from build123d import *

# Parameters (mm, degrees)
CROQUIS1_W              = 65.4
CROQUIS1_H              = 151.7
SALIENTE_EXTRUIR1_DEPTH = 93.8
CORTAR_EXTRUIR1_DEPTH   = 6
REDONDEO1_R             = 1
CORTAR_EXTRUIR2_DEPTH   = 1
CROQUIS4_W              = 14
CROQUIS4_H              = 16
CROQUIS4_W_2            = 13.98
CROQUIS4_H_2            = 15.98
CORTAR_EXTRUIR3_DEPTH   = 1
CROQUIS5_W              = 6.6
CROQUIS5_H              = 0.6
SALIENTE_EXTRUIR2_DEPTH = 4
CROQUIS6_W              = 6.6
CROQUIS6_H              = 0.5
SALIENTE_EXTRUIR3_DEPTH = 1
CROQUIS7_W              = 6
CROQUIS7_H              = 0.5
SALIENTE_EXTRUIR4_DEPTH = 6
REDONDEO2_R             = 0.5
CHAFL_N1_SIZE           = 1.5


with BuildPart() as part:
    # Croquis1 → Saliente-Extruir1 (new body)
    with BuildSketch(Plane(origin=(0, 0, 0), x_dir=(1, 0, 0), z_dir=(0, 1, 0))):
        Rectangle(CROQUIS1_W, CROQUIS1_H)
    extrude(amount=SALIENTE_EXTRUIR1_DEPTH)

    # Croquis2 → Cortar-Extruir1 (cut)
    with BuildSketch(Plane(origin=(0, 93.8, 0), x_dir=(1, 0, 0), z_dir=(0, 1, 0))):
        Polygon((-32.7, -56.85), (-32.7, 75.85), (32.7, 75.85), (32.7, -56.85), (31.2, -56.85), (31.2, 74.35), (-31.2, 74.35), (-31.2, -56.85), align=None)
    extrude(amount=-CORTAR_EXTRUIR1_DEPTH, mode=Mode.SUBTRACT)

    # Redondeo1
    redondeo1_edges = [part.edges().sort_by_distance(p)[0] for p in [
        (0, 93.8, 75.85),
        (-32.7, 93.8, 66.35),
        (-32.7, 43.9, -75.85),
        (32.7, 43.9, -75.85),
        (-32.7, 87.8, -9.5),
        (-32.7, 90.8, 56.85),
        (0, 87.8, -75.85),
        (32.7, 87.8, -9.5),
        (32.7, 90.8, 56.85),
        (31.2, 90.8, -74.35),
        (-31.2, 90.8, -74.35),
        (-31.95, 93.8, 56.85),
        (-31.2, 93.8, -8.75),
        (0, 93.8, -74.35),
        (31.2, 93.8, -8.75),
        (31.95, 93.8, 56.85),
        (32.7, 93.8, 66.35),
        (32.7, 46.9, 75.85),
        (-32.7, 46.9, 75.85),
    ]]
    fillet(redondeo1_edges, radius=REDONDEO1_R)

    # Croquis3 → Cortar-Extruir2 (cut)
    with BuildSketch(Plane(origin=(0, 93.8, 0), x_dir=(1, 0, 0), z_dir=(0, 1, 0))):
        with BuildLine():
            Line((-27.7, -53.85), (27.7, -53.85))
            ThreePointArc((27.7, -53.85), (28.407106781, -53.557106781), (28.7, -52.85))
            Line((28.7, -52.85), (28.7, 70.35))
            ThreePointArc((28.7, 70.35), (28.407106781, 71.057106781), (27.7, 71.35))
            Line((27.7, 71.35), (-27.7, 71.35))
            ThreePointArc((-27.7, 71.35), (-28.407106781, 71.057106781), (-28.7, 70.35))
            Line((-28.7, 70.35), (-28.7, -52.85))
            ThreePointArc((-28.7, -52.85), (-28.407106781, -53.557106781), (-27.7, -53.85))
        make_face()
        with BuildLine():
            Line((-26.7, -52.85), (26.7, -52.85))
            ThreePointArc((26.7, -52.85), (27.407106781, -52.557106781), (27.7, -51.85))
            Line((27.7, -51.85), (27.7, 69.35))
            ThreePointArc((27.7, 69.35), (27.407106781, 70.057106781), (26.7, 70.35))
            Line((26.7, 70.35), (-26.7, 70.35))
            ThreePointArc((-26.7, 70.35), (-27.407106781, 70.057106781), (-27.7, 69.35))
            Line((-27.7, 69.35), (-27.7, -51.85))
            ThreePointArc((-27.7, -51.85), (-27.407106781, -52.557106781), (-26.7, -52.85))
        make_face(mode=Mode.SUBTRACT)
    extrude(amount=-CORTAR_EXTRUIR2_DEPTH, mode=Mode.SUBTRACT)

    # Croquis4 → Cortar-Extruir3 (cut)
    # profile 1 of 2: a face of its own
    with BuildSketch(Plane(origin=(0, 93.8, 0), x_dir=(1, 0, 0), z_dir=(0, 1, 0))):
        with Locations((-22.2, -65.85)):
            Rectangle(CROQUIS4_W, CROQUIS4_H)
        with Locations((-22.2, -65.85)):
            Rectangle(CROQUIS4_W_2, CROQUIS4_H_2, mode=Mode.SUBTRACT)
    # profile 2 of 2: a face of its own
    with BuildSketch(Plane(origin=(0, 93.8, 0), x_dir=(1, 0, 0), z_dir=(0, 1, 0))):
        with Locations((22.2, -65.85)):
            Rectangle(CROQUIS4_W, CROQUIS4_H)
        with Locations((22.2, -65.85)):
            Rectangle(CROQUIS4_W_2, CROQUIS4_H_2, mode=Mode.SUBTRACT)
    extrude(amount=-CORTAR_EXTRUIR3_DEPTH, mode=Mode.SUBTRACT)

    # Croquis5 → Saliente-Extruir2 (add)
    with BuildSketch(Plane(origin=(0, 93.8, 0), x_dir=(1, 0, 0), z_dir=(0, 1, 0))):
        with Locations((-22.2, -59.16)):
            Rectangle(CROQUIS5_W, CROQUIS5_H)
        with Locations((22.2, -59.16)):
            Rectangle(CROQUIS5_W, CROQUIS5_H)
    extrude(amount=SALIENTE_EXTRUIR2_DEPTH)

    # Croquis6 → Saliente-Extruir3 (add)
    with BuildSketch(Plane(origin=(0, 0, 58.86), x_dir=(-1, 0, 0), z_dir=(0, 0, -1))):
        with Locations((22.2, 97.55)):
            Rectangle(CROQUIS6_W, CROQUIS6_H)
        with Locations((-22.2, 97.55)):
            Rectangle(CROQUIS6_W, CROQUIS6_H)
    extrude(amount=SALIENTE_EXTRUIR3_DEPTH)

    # Croquis7 → Saliente-Extruir4 (add)
    with BuildSketch(Plane(origin=(0, 0, 57.86), x_dir=(-1, 0, 0), z_dir=(0, 0, -1))):
        with Locations((22.2, 97.55)):
            Rectangle(CROQUIS7_W, CROQUIS7_H)
        with Locations((-22.2, 97.55)):
            Rectangle(CROQUIS7_W, CROQUIS7_H)
    extrude(amount=SALIENTE_EXTRUIR4_DEPTH)

    # Redondeo2
    redondeo2_edges = [part.edges().sort_by_distance(p)[0] for p in [
        (-22.2, 97.8, 59.46),
        (22.2, 97.8, 59.46),
        (-22.2, 97.3, 58.86),
        (22.2, 97.3, 58.86),
    ]]
    fillet(redondeo2_edges, radius=REDONDEO2_R)

    # Chaflán1
    chafl_n1_edges = [part.edges().sort_by_distance(p)[0] for p in [
        (-25.2, 97.55, 51.86),
        (-19.2, 97.55, 51.86),
        (25.2, 97.55, 51.86),
        (19.2, 97.55, 51.86),
    ]]
    chamfer(chafl_n1_edges, length=CHAFL_N1_SIZE)


solid = part.part
Design review of the part built by this model. Coordinates are the model's own, in mm. A direction names the side the tool comes from. Give positions to 0.01 mm unless a question says otherwise; leave off trailing zeros. Order: outer loops, then holes, each group sorted by start corner. A loop starts at its lowest first (then second) coordinate and runs counter-clockwise, first axis right, second up. Notation, with made-up numbers: (-12.75, 59) - (23.25, 59) arc R13 ccw to (23.25, 64) - close; hole circle Ø11 at (-10, 51.25). An arc over 180 degrees is marked (long way). Write item = value, one per line. Start each with the question number.
Q1. We need section C-C on x = -8. State the section outline as (y, z) points.
Q2. To check wall thickness, follow L1, parallel to Y at x = 23, z = 68; L2, parallel to X at y = 90.5, z = -24. State the ranges of each line that lie inside material, in increasing order. Write a range as from..to.
Q3. Tool access review of faces 1 (the face through (31.2, 90, -7)), 2 (the face through (0, 90, -74.35)), 3 (the face through (-22, 96, 59.46)), 4 (the face through (-31.2, 90, -9)), 5 (the face through (-22, 95, 58.86)): name each direction out of +Z, -Z, +X, -X, +Y, -Y from which nothing blocks a thin tool from reaching the whole face with its end or side.
Q4. We need section B-B on z = -36.5. State the section outline as (x, y) points.
Q5. We need section A-A on y = 90. State the section outline as (x, z) points.
Q6. Clearance check with flat-ended pins moving along their axes: pin 1 Ø11 at (x, z) = (-23, 65.5) entering from +Y; pin 2 Ø2.5 at (x, y) = (21.5, 94.5) entering from -Z; pin 3 Ø2.5 at (x, y) = (11.5, 89.5) entering from -Z. State where each tip first meets the part, or that it passes through.
Working result:
q1.outline = (0, -75.85) - (86.8, -75.85) arc R1 ccw to (87.8, -74.85) - (87.8, -74.35) - (92.8, -74.35) arc R1 ccw to (93.8, -73.35) - (93.8, -71.35) - (92.8, -71.35) - (92.8, -70.35) - (93.8, -70.35) - (93.8, 52.85) - (92.8, 52.85) - (92.8, 53.85) - (93.8, 53.85) - (93.8, 74.85) arc R1 ccw to (92.8, 75.85) - (0, 75.85) - close
q2.L1 = 0..93.8
q2.L2 = -31.2..31.2
q3.face_1 = -Z, +X, +Y
q3.face_2 = -Z, +X, -X, +Y
q3.face_3 = +Z, +X, -X, +Y
q3.face_4 = -Z, -X, +Y
q3.face_5 = -Z, +X, -X
q4.outline = (-32.7, 0) - (32.7, 0) - (32.7, 86.8) arc R1 ccw to (31.7, 87.8) - (31.2, 87.8) - (31.2, 92.8) arc R1 ccw to (30.2, 93.8) - (28.7, 93.8) - (28.7, 92.8) - (27.7, 92.8) - (27.7, 93.8) - (-27.7, 93.8) - (-27.7, 92.8) - (-28.7, 92.8) - (-28.7, 93.8) - (-30.2, 93.8) arc R1 ccw to (-31.2, 92.8) - (-31.2, 87.8) - (-31.7, 87.8) arc R1 ccw to (-32.7, 86.8) - close
q5.outline = (-32.7, 57.85) arc R1 ccw to (-31.7, 56.85) - (-31.2, 56.85) - (-31.2, -73.35) arc R1 ccw to (-30.2, -74.35) - (30.2, -74.35) arc R1 ccw to (31.2, -73.35) - (31.2, 56.85) - (31.7, 56.85) arc R1 ccw to (32.7, 57.85) - (32.7, 74.85) arc R1 ccw to (31.7, 75.85) - (-31.7, 75.85) arc R1 ccw to (-32.7, 74.85) - close
q6.pin_1 = 93.8
q6.pin_2 = -74.24
q6.pin_3 = -74.35
